Geometry check sheet. Reference: the model listing, model coordinates, mm. A direction names the side the tool comes from. Round coordinates to 2 decimals unless told otherwise and drop trailing zeros. Order: outer loops, then holes, each group sorted by start corner. A loop starts at its lowest first (then second) coordinate and runs counter-clockwise, first axis right, second up. Notation, with made-up numbers: (-7, -15) - (29, -15) arc R27 ccw to (29, 19) - close; hole circle Ø11 at (75.25, 1). An arc over 180 degrees is marked (long way). Use a Markdown table: item, result. Add a question column.
(1) Section check B-B on z = 10. Record the boundary of the cut face in (x, y).
(2) Thickness scan on line 1 along Y through (x, z) = (0, -4.15); line 2 along Z through (x, y) = (14, -6); line 3 along Z through (x, y) = (2.5, 10). Record the ranges inside material, lowest first. Write a range as [from, to].
(3) Access from +Z, -Z, +X, -X, +Y, -Y to the whole of each face (thin tool, end or side, straight path). Record for faces 4 (the face through (-4.302, -4.183, 5.916)), 5 (the face through (4.302, 4.183, 5.916)), 6 (the face through (-10.7, -15.8, -3.5)), 7 (the face through (-4.183, 4.302, 5.916)), 8 (the face through (6, -6, 0)).
(4) Mould release check, pull along X, two halves, no side actions. Record for faces 1 (the face through (-13, -12, -2)), 2 (the face through (4.183, -4.302, 5.916)), 3 (the face through (-0.65, -29.69, -2.46)): released by +X, released by -X, zero draft, split by the parting line, or undercut.
(5) Section check C-C on x = -20.5. Record the boundary of the cut face in (y, z), then the cut area to 3 significant figures.
(6) Section check A-A on y = 14.5. Record the boundary of the cut face in (x, z), then the cut area to 3 significant figures.
(7) Section check D-D on y = -15. Record the boundary of the cut face in (x, z).
(8) Gauge pin test, flat ends, axial feed: P1, Ø6, axis at x = 0.5, y = 18.5, coming from the +Z side; P2, Ø5, axis at x = 12.5, y = -11.5, coming from the -Z side; P3, Ø5, axis at y = 4.5, z = 4, coming from the -X side. Record the tip position at first contact, or that the pin passes through.
```python
from build123d import *

# Parameters (mm, degrees)
F2_DEPTH = 12
F4_DEPTH = 5
F5_R     = 4.75
F6_DEPTH = 3


with BuildPart() as f2:
    # F1 (on Top) → F2 (new body)
    with BuildSketch(Plane.XY):
        Polygon((-8.4852813742, 0), (0, -8.4852813742), (8.4852813742, 0), (0, 8.4852813742), align=None)
    extrude(amount=F2_DEPTH)

    # F3 (on Top) → F4 (join)
    with BuildSketch(Plane.XY):
        with BuildLine():
            Line((0, 29.6984848098), (-29.6984848098, 0))
            ThreePointArc((-29.6984848098, 0), (0, -29.6984848098), (29.6984848098, 0))
            Line((29.6984848098, 0), (0, 29.6984848098))
        make_face()
    extrude(amount=-F4_DEPTH)

    # F5 (on face) → F6 (cut)
    with BuildSketch(Plane(origin=(0, 0, -5), x_dir=(1, 0, 0), z_dir=(0, 0, -1))):
        with Locations((0, -11.6984848098)):
            Circle(F5_R)
        with Locations((-13.2155881356, 11.7721958357)):
            Circle(F5_R)
        with Locations((13.2155881356, 11.7721958357)):
            Circle(F5_R)
    extrude(amount=-F6_DEPTH, mode=Mode.SUBTRACT)


solid = f2.part
```
Check sheet entries:
| question | item | result |
|---|---|---|
| 1 | outline | (-8.49, 0) - (0, -8.49) - (8.49, 0) - (0, 8.49) - close |
| 2 | line 1 | y = [-29.7, 6.95], [16.45, 29.7] |
| 2 | line 2 | z = [-5, 0] |
| 2 | line 3 | z = [-2, 0] |
| 3 | face 4 | +Z, -X, -Y |
| 3 | face 5 | +Z, +X, +Y |
| 3 | face 6 | -Z |
| 3 | face 7 | +Z, -X, +Y |
| 3 | face 8 | +Z |
| 4 | face 1 | undercut |
| 4 | face 2 | released by +X |
| 4 | face 3 | split by the parting line |
| 5 | outline | (-21.49, -5) - (9.2, -5) - (9.2, 0) - (-21.49, 0) - close |
| 5 | area | 153 mm2 |
| 6 | outline | (-15.2, -5) - (-3.84, -5) - (-3.84, -2) - (3.84, -2) - (3.84, -5) - (15.2, -5) - (15.2, 0) - (-15.2, 0) - close |
| 6 | area | 129 mm2 |
| 7 | outline | (-25.63, -5) - (-16.7, -5) - (-16.7, -2) - (-9.73, -2) - (-9.73, -5) - (9.73, -5) - (9.73, -2) - (16.7, -2) - (16.7, -5) - (25.63, -5) - (25.63, 0) - (-25.63, 0) - close |
| 8 | P1 | stops at z = 0 |
| 8 | P2 | stops at z = -2 |
| 8 | P3 | stops at x = -6.49 |
